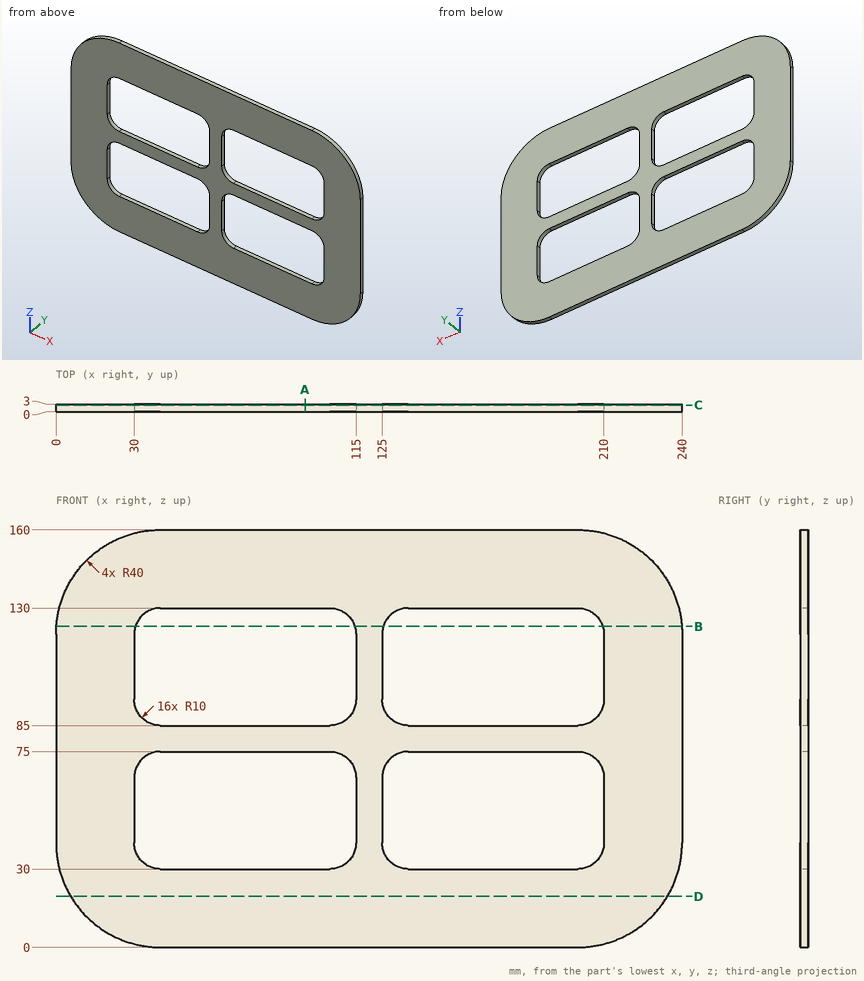
The drawing under review shows one solid part. Ordinate dimensions are in mm from its lowest x, y, z. Coordinates: 2 decimals unless noted, no trailing zeros. Write each loop counter-clockwise with the first axis right and the second up, starting at its lowest first coordinate (ties: lowest second). Pieces come first, ordered by that corner, then holes.
1) Add section C-C (y = 2.55). State how many separate pieces and enclosed holes the cut face has, plus the area to 3 significant figures.
2) Add section A-A (x = 95.5). Write out the cut boundary in (y, z), plus the area to 3 significant figures.
3) Add section D-D (z = 19.5). Write out the cut boundary in (x, y), plus the area to 3 significant figures.
4) Add section B-B (z = 123). Write out the cut boundary in (x, y).
5) To check wall thickness, follow L1, parallel to X at y = 1.85, z = 49; L2, parallel to Z at x = 164, y = 2.4; L3, parallel to X at y = 2.75, z = 69. State the ranges of each line that lie inside material, in increasing order.
Check result:
1. separate pieces: 1
1. enclosed holes: 4
1. area: 22,100 mm2
2. outline: (0, 0) - (3, 0) - (3, 30) - (0, 30) - close; (0, 75) - (3, 75) - (3, 85) - (0, 85) - close; (0, 130) - (3, 130) - (3, 160) - (0, 160) - close
2. area: 210 mm2
3. outline: (5.65, 0) - (234.35, 0) - (234.35, 3) - (5.65, 3) - close
3. area: 686 mm2
4. outline: (0.11, 0) - (30.46, 0) - (30.46, 3) - (0.11, 3) - close; (114.54, 0) - (125.46, 0) - (125.46, 3) - (114.54, 3) - close; (209.54, 0) - (239.89, 0) - (239.89, 3) - (209.54, 3) - close
5. L1: x = 0 to 30, 115 to 125, 210 to 240
5. L2: z = 0 to 30, 75 to 85, 130 to 160
5. L3: x = 0 to 30.83, 114.17 to 125.83, 209.17 to 240
